Input: part model. Units: mm. Frame: model coordinates. Give positions to 0.01 mm unless a question says otherwise; leave off trailing zeros. Loops run counter-clockwise (first coordinate to the right, second up) from the corner with the lowest first, then second, coordinate; pieces in that order, holes last. Notation, with made-up numbers: (76.5, 3) -> (92.5, 3) arc R24 cw to (92.5, 14) -> close; hole circle Ø11 at (1, 71.25). An arc over 180 degrees is marked (long way). Answer in a Markdown table with one row per item. Add a question column.
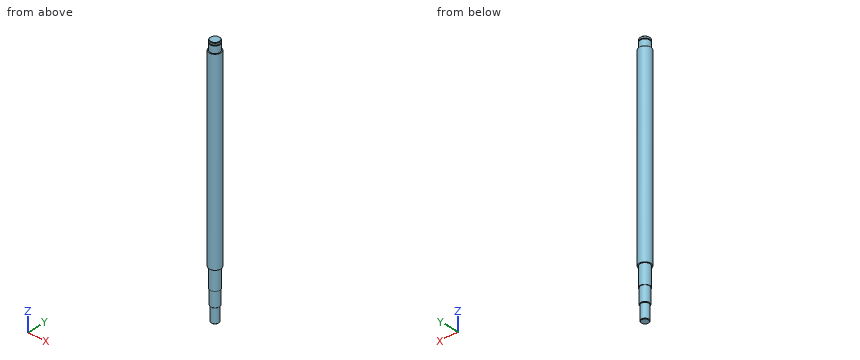
```python
from build123d import *


with BuildPart() as f1:
    # F0 (on Front) → F1 (revolve)
    with BuildSketch(Plane.XZ):
        Polygon((0, 260), (0, 0), (3.5, 0), (4, 0.5), (4, 15), (4.5, 15.5), (4.5, 31), (5, 31), (5, 51), (6, 51), (6, 250), (5, 250), (5, 257), (3.8, 257), (3.8, 257.9), (5, 257.9), (5, 259.5), (4.5, 260), align=None)
    revolve(axis=Axis((0, 0, 142.919585), (0, 0, 1)))


solid = f1.part
```
1) Section C-C on z = 45.5. Output: boundary loops of the cut face in (x, y), and give its area (3 significant figures).
2) Material intervals for line 1 along Z through (x, y) = (2.5, -4.75); line 2 along Y through (x, z) = (-0.75, 100); line 3 along X through (y, z) = (-4.5, 150), sorted ascending.
3) Pin query (flat end, axial travel): pin 1 (1.5 mm diameter, centred on x = -2, z = 208, fed in from -Y); pin 2 (1 mm diameter, centred on x = 4, z = 152.5, fed in from -Y). Return the tip coordinate at first contact, or that it passes through.
4) Section D-D on z = 223. Output: boundary loops of the cut face in (x, y), and give its area (3 significant figures).
Working result:
| question | item | result |
|---|---|---|
| 1 | outline | circle Ø10 at (0, 0) |
| 1 | area | 78.5 mm2 |
| 2 | line 1 | z = 51 to 250 |
| 2 | line 2 | y = -5.95 to 5.95 |
| 2 | line 3 | x = -3.97 to 3.97 |
| 3 | pin 1 | stops at y = -5.87 |
| 3 | pin 2 | stops at y = -4.87 |
| 4 | outline | circle Ø12 at (0, 0) |
| 4 | area | 113 mm2 |
